Geometry: see drawing. Coordinates: mm, zero at the bounding-box minimum. Coordinates: 2 decimals unless noted, no trailing zeros. Loops run counter-clockwise (first coordinate to the right, second up) from the corner with the lowest first, then second, coordinate; pieces in that order, holes last. Notation, with made-up numbers: (31, 46.25) - (86, 46.25) arc R27 ccw to (86, 71.25) - close; hole circle Ø4 at (31, 56.25). An arc over 180 degrees is marked (long way). Use a Markdown table: item, result. Add a question column.
1. Section query A-A on x = 12. Return the cut outline in (y, z).
2. Section query B-B on z = 12. Return the cut outline in (x, y).
3. Section query C-C on y = 2.8. Return the cut outline in (x, z), then the cut area to 3 significant figures.
4. Draft query along X for the marked faces 1, 2 and 3. Return one class per face: released by +X, released by -X, zero draft, split by the parting line, or undercut.
5. Section query D-D on y = 4.35. Return the cut outline in (x, z), then the cut area to 3 significant figures.
6. Contact query for flat-ended pins moving along their axis: P1, Ø1, axis at x = 12, y = 2.5, coming from the +Z side; P2, Ø5, axis at x = 17.5, z = 7.5, coming from the +Y side; P3, Ø2, axis at x = 6, z = 10.5, coming from the +Y side. Output: stop coordinate, or through.
7. Ray query, L1, parallel to Z at x = 12, y = 1.45; L2, parallel to Y at x = 6.5, z = 3.25; L3, parallel to Z at x = 17.75, y = 4.4. Return the intervals inside material, ascending. Write a range as [from, to].
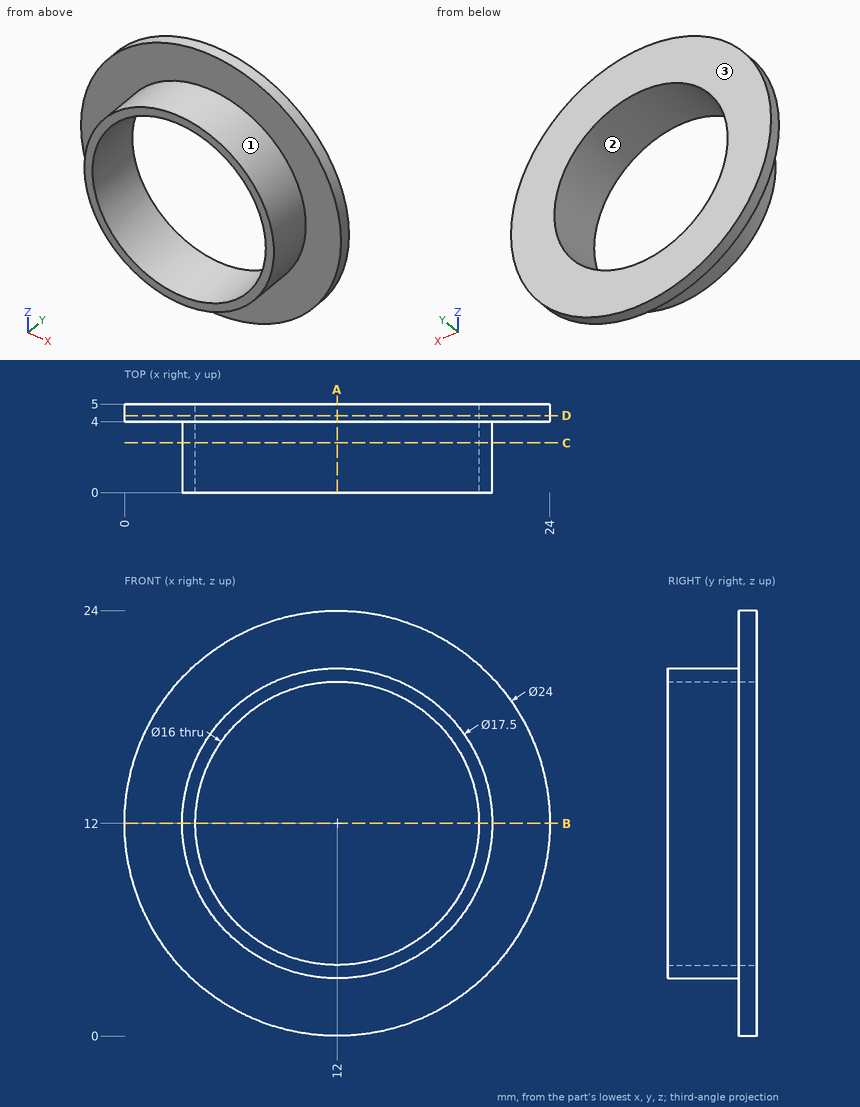
Resolved:
| question | item | result |
|---|---|---|
| 1 | outline | (0, 3.25) - (4, 3.25) - (4, 0) - (5, 0) - (5, 4) - (0, 4) - close; (0, 20) - (5, 20) - (5, 24) - (4, 24) - (4, 20.75) - (0, 20.75) - close |
| 2 | outline | (0, 4) - (3.25, 4) - (3.25, 0) - (4, 0) - (4, 5) - (0, 5) - close; (20, 0) - (20.75, 0) - (20.75, 4) - (24, 4) - (24, 5) - (20, 5) - close |
| 3 | outline | circle Ø17.5 at (12, 12); hole circle Ø16 at (12, 12) |
| 3 | area | 39.5 mm² |
| 4 | face 1 | split by the parting line |
| 4 | face 2 | undercut |
| 4 | face 3 | zero draft |
| 5 | outline | circle Ø24 at (12, 12); hole circle Ø16 at (12, 12) |
| 5 | area | 251 mm² |
| 6 | P1 | z = 20.75 |
| 6 | P2 | y = 5 |
| 6 | P3 | through |
| 7 | L1 | [3.25, 4], [20, 20.75] |
| 7 | L2 | [4, 5] |
| 7 | L3 | [1.47, 6.44], [17.56, 22.53] |
